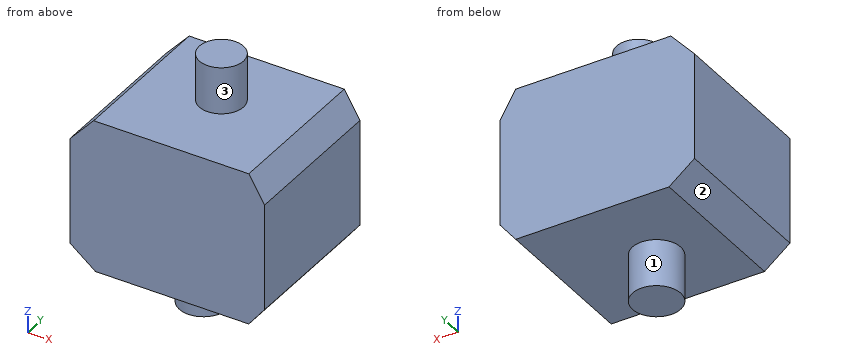
from build123d import *

# Parameters (mm, degrees)
F1_DEPTH = 101.6
F2_R     = 14.570657
F3_DEPTH = 30.988
F4_R     = 15.889172
F5_DEPTH = 30.988


with BuildPart() as f1:
    # F0 (on Front) → F1 (new body)
    with BuildSketch(Plane.XZ):
        Polygon((58.653947, 47.223948), (-43.915264, 47.223948), (-59.556317, 29.778158), (-59.556317, -40.606577), (-42.712107, -53.841315), (58.653947, -53.841315), (69.052672, -40.606577), (69.052672, 29.778158), align=None)
    extrude(amount=F1_DEPTH)

    # F2 (on face) → F3 (join)
    with BuildSketch(Plane.XY.offset(47.223948)):
        with Locations((5.683666, -45.478929)):
            Circle(F2_R)
    extrude(amount=F3_DEPTH)

    # F4 (on face) → F5 (join)
    with BuildSketch(Plane(origin=(0, 0, -53.841315), x_dir=(1, 0, 0), z_dir=(0, 0, -1))):
        with Locations((0, 55.446912)):
            Circle(F4_R)
    extrude(amount=F5_DEPTH)


solid = f1.part
Could you check a few things on this model? Use its own coordinates, in mm. Face numbers are marked on the shaded views. A direction names the side the tool comes from. Round coordinates to 2 decimals unless told otherwise and drop trailing zeros. Write each loop counter-clockwise with the first axis right and the second up, starting at its lowest first coordinate (ties: lowest second). Pieces come first, ordered by that corner, then holes. Notation, with made-up numbers: (50.5, 29) -> (87.5, 29) arc R22 ccw to (87.5, 59) -> close; hole circle Ø1 at (41.25, 59.25). An arc over 180 degrees is marked (long way). Use a Markdown table: item, result.
1. Which directions (+Z, -Z, +X, -X, +Y, -Y) give clear straight access to the entire face, cutting with the end or side of a thin tool? Please do the marked faces 1, 2 and 3.
Answer key:
| item | result |
|---|---|
| face 1 | -Z |
| face 2 | -Z, -X, +Y, -Y |
| face 3 | +Z |
2. For pin 1 Ø6 at (x, y) = (-30.5, -75) entering from -Z; pin 2 Ø1 at (x, z) = (24.5, -12.5) entering from +Y; pin 3 Ø1 at (x, y) = (47.5, -19) entering from +Z; pin 4 Ø2 at (x, z) = (17, 52.5) entering from -Y, each with a flat end and sliding along its axis, tell me the tip position at first contact or that it passes through.
Answer key:
| item | result |
|---|---|
| pin 1 | stops at z = -53.84 |
| pin 2 | stops at y = 0 |
| pin 3 | stops at z = 47.22 |
| pin 4 | stops at y = -55.77 |
3. If we section it at C-C (y = -67): List the corners of the cut face in (x, z) for me, then the cut area to 3 significant figures.
Answer key:
| item | result |
|---|---|
| outline | (-59.56, -40.61) -> (-42.71, -53.84) -> (-10.91, -53.84) -> (-10.91, -84.83) -> (10.91, -84.83) -> (10.91, -53.84) -> (58.65, -53.84) -> (69.05, -40.61) -> (69.05, 29.78) -> (58.65, 47.22) -> (-43.92, 47.22) -> (-59.56, 29.78) -> close |
| area | 13,300 mm^2 |
4. If we section it at B-B (x = -5): List the corners of the cut face in (y, z) for me.
Answer key:
| item | result |
|---|---|
| outline | (-101.6, -53.84) -> (-70.53, -53.84) -> (-70.53, -84.83) -> (-40.36, -84.83) -> (-40.36, -53.84) -> (0, -53.84) -> (0, 47.22) -> (-35.57, 47.22) -> (-35.57, 78.21) -> (-55.39, 78.21) -> (-55.39, 47.22) -> (-101.6, 47.22) -> close |
5. If we section it at A-A (y = -15.5): List the corners of the cut face in (x, z) for me, then the cut area to 3 significant figures.
Answer key:
| item | result |
|---|---|
| outline | (-59.56, -40.61) -> (-42.71, -53.84) -> (58.65, -53.84) -> (69.05, -40.61) -> (69.05, 29.78) -> (58.65, 47.22) -> (-43.92, 47.22) -> (-59.56, 29.78) -> close |
| area | 12,600 mm^2 |
6. If we section it at D-D (z = 44.5): List the corners of the cut face in (x, y) for me, then the cut area to 3 significant figures.
Answer key:
| item | result |
|---|---|
| outline | (-46.36, -101.6) -> (60.28, -101.6) -> (60.28, 0) -> (-46.36, 0) -> close |
| area | 10,800 mm^2 |
7. Please list where these lines run through material, in increasing order: probe 1 along Z at (x, y) = (38, -52); probe 2 along Z at (x, y) = (-6, -56); probe 3 along X at (y, z) = (-80.5, 44.5).
Answer key:
| item | result |
|---|---|
| probe 1 | z = -53.84 to 47.22 |
| probe 2 | z = -84.83 to 47.22 |
| probe 3 | x = -46.36 to 60.28 |
